from build123d import *

# Parameters (mm, degrees)
BOSS_EXTRUDE1_DEPTH      = 3
BOSS_EXTRUDE1_DEPTH_BACK = 6
SKETCH1_R                = 10
SKETCH4_R                = 1.6
HOLE_DEPTH               = 19.539009706
HOLECIR_COUNT            = 5
FILLET3_R                = 2
BOSS_EXTRUDE2_START      = 8.5
SKETCH5_R                = 10
BOSS_EXTRUDE2_DEPTH      = 8.5
SKETCH6_R                = 2
CUT_EXTRUDE1_DEPTH       = 11.1


with BuildPart() as part:
    # Sketch1 → Boss-Extrude1 (new, two sides: drawn at the far end of the back side and taken through both)
    with BuildSketch(Plane(origin=(0, 0, 0), x_dir=(1, 0, 0), z_dir=(0, 1, 0)).offset(-BOSS_EXTRUDE1_DEPTH_BACK)):
        with Locations(Location((0, 0, 0), (0, 0, 270))):
            Circle(SKETCH1_R)
    extrude(amount=BOSS_EXTRUDE1_DEPTH + BOSS_EXTRUDE1_DEPTH_BACK)

    # Sketch4 → hole (cut, through all)
    with BuildSketch(Plane(origin=(-3.352872105, -1.093066116, 1.887711608), x_dir=(-0.4486862613641547, -0.14627571033740308, -0.8816371449912632), z_dir=(0.8382180262940947, 0.2732665289126682, -0.47192790187872385))):
        with Locations(Location((0, 0, 0), (0, 0, 8.746528197))):
            Circle(SKETCH4_R)
    hole = extrude(amount=-HOLE_DEPTH, mode=Mode.SUBTRACT)

    # holecir: hole ×5 about axis
    holecir_axis = Axis((0, 0, 0), (0, 1, 0))
    for i in range(1, HOLECIR_COUNT):
        add(hole.rotate(holecir_axis, i * 360 / HOLECIR_COUNT), mode=Mode.SUBTRACT)

    # Fillet3
    fillet3_edges = [part.edges().sort_by_distance(p)[0] for p in [
        (0, 3, -10),
    ]]
    fillet(fillet3_edges, radius=FILLET3_R)

    # Sketch5 → Boss-Extrude2 (add)
    with BuildSketch(Plane.XZ.offset(6).offset(BOSS_EXTRUDE2_START)):
        with Locations(Location((0, 0, 0), (0, 0, 90))):
            Circle(SKETCH5_R)
    extrude(amount=-BOSS_EXTRUDE2_DEPTH)

    # Sketch6 → Cut-Extrude1 (cut)
    with BuildSketch(Plane.XZ.offset(14.5)):
        with Locations(Location((0, 0, 0), (0, 0, 270))):
            Circle(SKETCH6_R)
    extrude(amount=-CUT_EXTRUDE1_DEPTH, mode=Mode.SUBTRACT)


solid = part.part
Geometry check sheet. Reference: the model listing, model coordinates, mm. A direction names the side the tool comes from. Coordinates: 2 decimals unless noted, no trailing zeros. Loops run counter-clockwise (first coordinate to the right, second up) from the corner with the lowest first, then second, coordinate; pieces in that order, holes last. Notation, with made-up numbers: (7, 55) - (54, 55) arc R19 ccw to (54, 60) - close; hole circle Ø1 at (4, -11.5). An arc over 180 degrees is marked (long way). Use one line per item in the form item = value. Start each with the question number.
Item 1: Mould release check, pull along Y, two halves, no side actions. Record for faces 1 (the face through (-5.14, -3.52, -4.26)), 2 (the face through (-2, -9, 0)), 3 (the face through (-2.4, -14.5, -0.1)): +Y half, -Y half, draft (parallel to the pull), parting line (faces both ways), or undercut.
Item 2: Section check B-B, the plane x = -3.5. Give the number of separate pieces and of enclosed holes in the cut face, and give its area (3 significant figures).
Item 3: Tool access check on faces 4 (the face through (0, -3.4, 0)), 5 (the face through (0, 3, 0)), 6 (the face through (-3.35, -1.07, 1.91)). Record the directions out of +Z, -Z, +X, -X, +Y, -Y that give a thin tool (end or side, any length) a straight path to the whole face; none if there is none.
Item 4: Gauge pin test, flat end, axial feed: pin 1 (6 mm diameter, centred on y = -10.5, z = 3.5, fed in from +X). Record the tip position at first contact, or that the pin passes through.
Item 5: Section check D-D, the plane y = 2.25. Enter the section's corners in (x, z), and give its area (3 significant figures).
Item 6: Thickness scan on probe 1 along X at (y, z) = (-7, 0); probe 2 along Z at (x, y) = (0.5, -0.75); probe 3 along Z at (x, y) = (0.75, -7.75). Record the ranges inside material, lowest first.
Item 7: Section check A-A, the plane y = -11. Enter the section's corners in (x, z).
Computed:
q1.face_1 = undercut
q1.face_2 = draft
q1.face_3 = -Y half
q2.separate_pieces = 1
q2.enclosed_holes = 2
q2.area = 310 mm2
q3.face_4 = -Y
q3.face_5 = +Z, -Z, +X, -X, +Y
q3.face_6 = none
q4.pin_1 = 9.99
q5.outline = circle Ø19.12 at (0, 0)
q5.area = 287 mm2
q6.probe_1 = -10 to -2, 2 to 10
q6.probe_2 = -9.99 to -4.73, -4.11 to 3.92, 7.36 to 9.99
q6.probe_3 = -9.97 to -1.85, 1.85 to 9.97
q7.outline = circle Ø20 at (0, 0); hole circle Ø4 at (0, 0)
